```python
from build123d import *

# Parameters (mm, degrees)
SKETCH1_W               = 121.5
SKETCH1_H               = 52
BOSS_EXTRUDE1_DEPTH     = 6
CHAMFER1_SIZE           = 20
M5_CLEARANCE_HOLE1_D    = 5.3
CUT_EXTRUDE4_DEPTH      = 7
M3_CLEARANCE_HOLE1_D    = 3.2
SKETCH6_R               = 11
CUT_EXTRUDE3_DEPTH      = 7
SKETCH234_W             = 10
SKETCH234_H             = 6
BOSS_EXTRUDE234_DEPTH   = 6
FILLET134_R             = 1
SKETCH2341_W            = 10
SKETCH2341_H            = 6
BOSS_EXTRUDE2341_DEPTH  = 6
FILLET1341_R            = 1
SKETCH2342_W            = 10
SKETCH2342_H            = 6
BOSS_EXTRUDE2342_DEPTH  = 6
FILLET1342_R            = 1
SKETCH2343_W            = 10
SKETCH2343_H            = 6
BOSS_EXTRUDE2343_DEPTH  = 6
FILLET1343_R            = 1
SKETCH2345_W            = 10
SKETCH2345_H            = 6
BOSS_EXTRUDE2345_DEPTH  = 6
FILLET1345_R            = 1
SKETCH2346_W            = 10
SKETCH2346_H            = 6
BOSS_EXTRUDE2346_DEPTH  = 6
FILLET1346_R            = 1
FILLET1347_R            = 10
SKETCH62_W              = 10
SKETCH62_H              = 6
CUT_EXTRUDE1_DEPTH      = 4
CUT_EXTRUDE1_DEPTH_BACK = 4


with BuildPart() as part:
    # Sketch1 → Boss-Extrude1 (new body)
    with BuildSketch(Plane(origin=(0, 0, 0), x_dir=(1, 0, 0), z_dir=(0, 1, 0))):
        with Locations((60.75, 26)):
            Rectangle(SKETCH1_W, SKETCH1_H)
    extrude(amount=BOSS_EXTRUDE1_DEPTH)

    # Chamfer1
    chamfer1_edges = [part.edges().sort_by_distance(p)[0] for p in [
        (121.5, 3, -52),
    ]]
    chamfer(chamfer1_edges, length=CHAMFER1_SIZE)

    # M5 Clearance Hole1 (through all)
    with Locations(Plane(origin=(0, 6, 0), x_dir=(1, 0, 0), z_dir=(0, 1, 0))):
        with Locations((111.5, 26)):
            Hole(M5_CLEARANCE_HOLE1_D / 2)

    # Sketch7 → Cut-Extrude4 (cut, through all)
    with BuildSketch(Plane(origin=(0, 6, 0), x_dir=(1, 0, 0), z_dir=(0, 1, 0))):
        with BuildLine():
            Line((56.5, 44.65), (96.5, 44.65))
            ThreePointArc((96.5, 44.65), (99.15, 42), (96.5, 39.35))
            Line((96.5, 39.35), (56.5, 39.35))
            ThreePointArc((56.5, 39.35), (53.85, 42), (56.5, 44.65))
        make_face()
    extrude(amount=-CUT_EXTRUDE4_DEPTH, mode=Mode.SUBTRACT)

    # M3 Clearance Hole1 (through all)
    with Locations(Plane(origin=(26, 0, -26), x_dir=(0, 0, 1), z_dir=(0, -1, 0))):
        with Locations((15.5, -15.5), (-15.5, -15.5), (-15.5, 15.5), (15.5, 15.5)):
            Hole(M3_CLEARANCE_HOLE1_D / 2)

    # Sketch6 → Cut-Extrude3 (cut, through all)
    with BuildSketch(Plane(origin=(26, 0, -26), x_dir=(0, 0, -1), z_dir=(0, -1, 0))):
        Circle(SKETCH6_R)
    extrude(amount=-CUT_EXTRUDE3_DEPTH, mode=Mode.SUBTRACT)

    # Sketch234 → Boss-Extrude234 (add)
    with BuildSketch(Plane(origin=(16.767778608, 6, 0), x_dir=(-1, 0, 0), z_dir=(0, 0, 1))):
        with Locations((0.767778608, 3)):
            Rectangle(SKETCH234_W, SKETCH234_H)
    extrude(amount=BOSS_EXTRUDE234_DEPTH)

    # Fillet134
    fillet134_edges = [part.edges().sort_by_distance(p)[0] for p in [
        (21, 3, 6),
        (11, 3, 6),
    ]]
    fillet(fillet134_edges, radius=FILLET134_R)

    # Sketch2341 → Boss-Extrude2341 (add)
    with BuildSketch(Plane(origin=(46.601111941, 6, 0), x_dir=(-1, 0, 0), z_dir=(0, 0, 1))):
        with Locations((0.767778608, 3)):
            Rectangle(SKETCH2341_W, SKETCH2341_H)
    extrude(amount=BOSS_EXTRUDE2341_DEPTH)

    # Fillet1341
    fillet1341_edges = [part.edges().sort_by_distance(p)[0] for p in [
        (40.833333333, 3, 6),
        (50.833333333, 3, 6),
    ]]
    fillet(fillet1341_edges, radius=FILLET1341_R)

    # Sketch2342 → Boss-Extrude2342 (add)
    with BuildSketch(Plane(origin=(76.434445274, 6, 0), x_dir=(-1, 0, 0), z_dir=(0, 0, 1))):
        with Locations((0.767778608, 3)):
            Rectangle(SKETCH2342_W, SKETCH2342_H)
    extrude(amount=BOSS_EXTRUDE2342_DEPTH)

    # Fillet1342
    fillet1342_edges = [part.edges().sort_by_distance(p)[0] for p in [
        (70.666666667, 3, 6),
        (80.666666667, 3, 6),
    ]]
    fillet(fillet1342_edges, radius=FILLET1342_R)

    # Sketch2343 → Boss-Extrude2343 (add)
    with BuildSketch(Plane(origin=(106.267778608, 6, 0), x_dir=(-1, 0, 0), z_dir=(0, 0, 1))):
        with Locations((0.767778608, 3)):
            Rectangle(SKETCH2343_W, SKETCH2343_H)
    extrude(amount=BOSS_EXTRUDE2343_DEPTH)

    # Fillet1343
    fillet1343_edges = [part.edges().sort_by_distance(p)[0] for p in [
        (100.5, 3, 6),
        (110.5, 3, 6),
    ]]
    fillet(fillet1343_edges, radius=FILLET1343_R)

    # Sketch2345 → Boss-Extrude2345 (add)
    with BuildSketch(Plane(origin=(0, 0, -15.767778608), x_dir=(0, 0, 1), z_dir=(-1, 0, 0))):
        with Locations((0.767778608, 3)):
            Rectangle(SKETCH2345_W, SKETCH2345_H)
    extrude(amount=BOSS_EXTRUDE2345_DEPTH)

    # Fillet1345
    fillet1345_edges = [part.edges().sort_by_distance(p)[0] for p in [
        (-6, 3, -20),
        (-6, 3, -10),
    ]]
    fillet(fillet1345_edges, radius=FILLET1345_R)

    # Sketch2346 → Boss-Extrude2346 (add)
    with BuildSketch(Plane(origin=(0, 6, -39.232221392), x_dir=(0, 0, -1), z_dir=(-1, 0, 0))):
        with Locations((0.767778608, 3)):
            Rectangle(SKETCH2346_W, SKETCH2346_H)
    extrude(amount=BOSS_EXTRUDE2346_DEPTH)

    # Fillet1346
    fillet1346_edges = [part.edges().sort_by_distance(p)[0] for p in [
        (-6, 3, -45),
        (-6, 3, -35),
    ]]
    fillet(fillet1346_edges, radius=FILLET1346_R)

    # Fillet1347
    fillet1347_edges = [part.edges().sort_by_distance(p)[0] for p in [
        (101.5, 3, -52),
        (121.5, 3, -32),
    ]]
    fillet(fillet1347_edges, radius=FILLET1347_R)

    # Sketch62 → Cut-Extrude1 (cut, two sides)
    with BuildSketch(Plane(origin=(66.5, 3, -10.767778608), x_dir=(0, 0, 1), z_dir=(0, -1, 0))) as cut_extrude1_sk:
        with Locations((0.767778608, -44)):
            Rectangle(SKETCH62_W, SKETCH62_H)
    extrude(amount=CUT_EXTRUDE1_DEPTH, mode=Mode.SUBTRACT)
    extrude(cut_extrude1_sk.sketch, amount=-CUT_EXTRUDE1_DEPTH_BACK, mode=Mode.SUBTRACT)


solid = part.part
```
Input: part model. Units: mm. Frame: model coordinates. A direction names the side the tool comes from. Coordinates: 2 decimals unless noted, no trailing zeros. Loops run counter-clockwise (first coordinate to the right, second up) from the corner with the lowest first, then second, coordinate; pieces in that order, holes last. Notation, with made-up numbers: M 21.5,14 L 47.5,14 A24 cw 47.5,24 Z; hole C 25.25,-0.5 d4. An arc over 180 degrees is marked long. Use a Markdown table: item, result. Add a question column.
1) Pin query (flat end, axial travel): P1, Ø3, axis at x = 32, y = 4, coming from the +Z side; P2, Ø1.5, axis at y = 1, z = -31, coming from the +X side; P3, Ø3, axis at x = 70, y = 4, coming from the +Z side. Return the tip coordinate at first contact, or that it passes through.
2) Draft query along Z for faces 1 (the flat face through (121.5, 3, -14)), 2 (the flat face through (-2, 3, -35)), 3 (the flat face through (48, 3, -52)). Return one class per face: +Z half, -Z half, draft (parallel to the pull), parting line (faces both ways), or undercut.
3) Section B-B, the plane z = -26. Return the cut outline in (x, y), plus the area to 3 significant figures.
4) Section C-C, the plane y = 1.5. Give the number of separate pieces and of enclosed holes in the cut face, plus the area to 3 significant figures.
5) Line query: L1, parallel to Z at x = 72, y = 5.5; L2, parallel to Z at x = 111.5, y = 1.5; L3, parallel to Z at x = 41.5, y = 2.7. Output: solid intervals per line, ascending. Write a range as from..to.
6) Section A-A, the plane x = 26. Return the cut outline in (y, z), plus the area to 3 significant figures.
7) Section D-D, the plane x = 86. Return the cut outline in (y, z), plus the area to 3 significant figures.
8) Set-up query: faces 4 (the flat face through (0, 3, -27)), 5 (the flat face through (110.5, 3, 2)), 6 (the flat face through (90, 3, 0)), 7 (the flat face through (11, 3, 2)), 8 (the flat face through (0, 3, -48)). Return all of +Z, -Z, +X, -X, +Y, -Y with unobstructed straight access to the full face (end or side cutting, diameter ignored); none if empty.
Answer below:
| question | item | result |
|---|---|---|
| 1 | P1 | z = 0 |
| 1 | P2 | x = 121.21 |
| 1 | P3 | z = 5.99 |
| 2 | face 1 | draft |
| 2 | face 2 | undercut |
| 2 | face 3 | -Z half |
| 3 | outline | M 0,0 L 15,0 L 15,6 L 0,6 Z; M 37,0 L 108.85,0 L 108.85,6 L 37,6 Z; M 114.15,0 L 121.5,0 L 121.5,6 L 114.15,6 Z |
| 3 | area | 565 mm2 |
| 4 | separate pieces | 1 |
| 4 | enclosed holes | 8 |
| 4 | area | 5,740 mm2 |
| 5 | L1 | -52..-44.65, -39.35..6 |
| 5 | L2 | -42..-28.65, -23.35..-15, -5..0 |
| 5 | L3 | -52..-43.1, -39.9..-12.1, -8.9..5.94 |
| 6 | outline | M 0,-52 L 6,-52 L 6,-37 L 0,-37 Z; M 0,-15 L 6,-15 L 6,0 L 0,0 Z |
| 6 | area | 180 mm2 |
| 7 | outline | M 0,-52 L 6,-52 L 6,-44.65 L 0,-44.65 Z; M 0,-39.35 L 6,-39.35 L 6,0 L 0,0 Z |
| 7 | area | 280 mm2 |
| 8 | face 4 | -X, +Y, -Y |
| 8 | face 5 | +Z, +X, +Y, -Y |
| 8 | face 6 | +Z, +Y, -Y |
| 8 | face 7 | +Z, -X, +Y, -Y |
| 8 | face 8 | -Z, -X, +Y, -Y |
